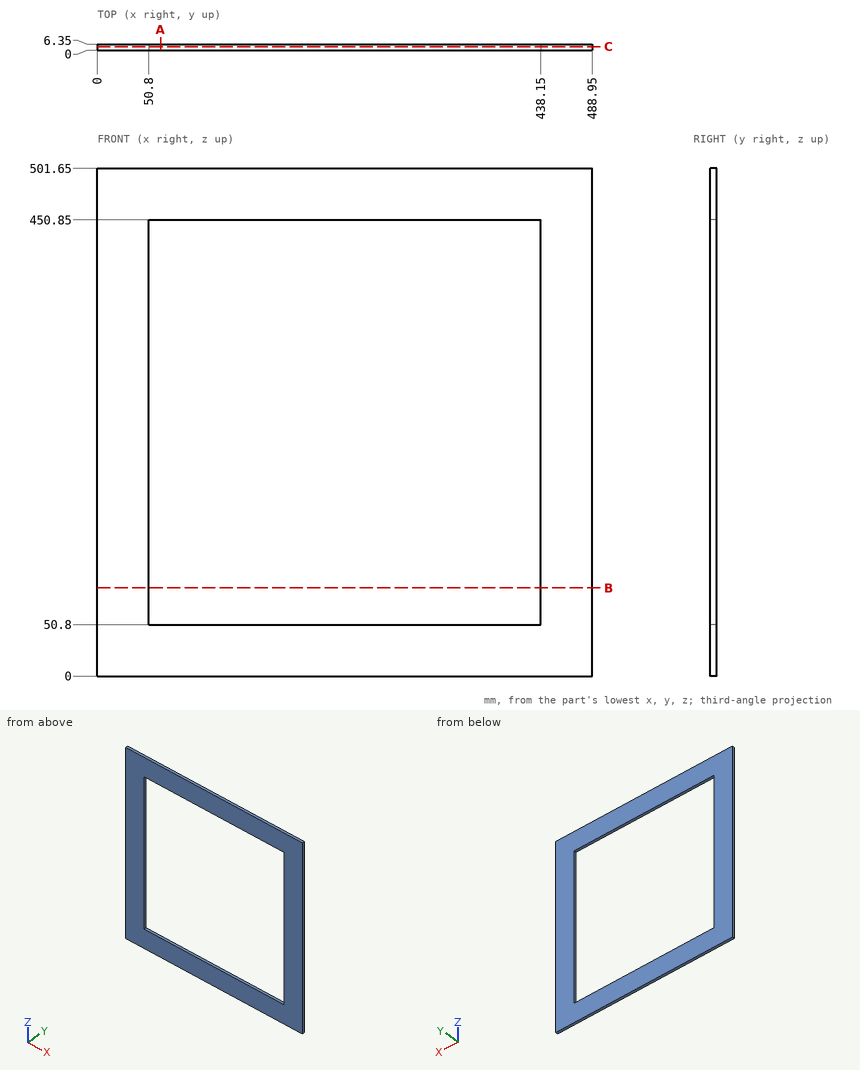
Geometry: see drawing. Coordinates: mm, zero at the bounding-box minimum. Coordinates: 2 decimals unless noted, no trailing zeros. Loops run counter-clockwise (first coordinate to the right, second up) from the corner with the lowest first, then second, coordinate; pieces in that order, holes last. Notation, with made-up numbers: (73, 5.25) -> (108, 5.25) arc R13 ccw to (108, 10.25) -> close; hole circle Ø7 at (33, -19.5). An arc over 180 degrees is marked (long way). Use a Markdown table: item, result.
1) Cut plane C-C (y = 3.75). Return the cut outline in (x, z), then the cut area to 3 significant figures.
Results found:
| item | result |
|---|---|
| outline | (0, 0) -> (488.95, 0) -> (488.95, 501.65) -> (0, 501.65) -> close; hole (50.8, 50.8) -> (438.15, 50.8) -> (438.15, 450.85) -> (50.8, 450.85) -> close |
| area | 90,300 mm2 |
2) Material intervals for line 1 along Z through (x, y) = (225.5, 3.25); line 2 along X through (y, z) = (2, 388), sorted ascending. Write a range as from..to.
Results found:
| item | result |
|---|---|
| line 1 | z = 0..50.8, 450.85..501.65 |
| line 2 | x = 0..50.8, 438.15..488.95 |
3) Cut plane A-A (x = 62.5). Return the cut outline in (y, z), then the cut area to 3 significant figures.
Results found:
| item | result |
|---|---|
| outline | (0, 0) -> (6.35, 0) -> (6.35, 50.8) -> (0, 50.8) -> close; (0, 450.85) -> (6.35, 450.85) -> (6.35, 501.65) -> (0, 501.65) -> close |
| area | 645 mm2 |
4) Cut plane B-B (z = 87). Return the cut outline in (x, y), then the cut area to 3 significant figures.
Results found:
| item | result |
|---|---|
| outline | (0, 0) -> (50.8, 0) -> (50.8, 6.35) -> (0, 6.35) -> close; (438.15, 0) -> (488.95, 0) -> (488.95, 6.35) -> (438.15, 6.35) -> close |
| area | 645 mm2 |
